```python
from build123d import *

# Parameters (mm, degrees)
CROQUIS1_W              = 192.96
CROQUIS1_H              = 110.76
CROQUIS1_W_2            = 172.96
CROQUIS1_H_2            = 102.76
SALIENTE_EXTRUIR2_DEPTH = 18
CROQUIS2_W              = 31.89
CROQUIS2_H              = 3
SALIENTE_EXTRUIR3_DEPTH = 24.43
CROQUIS3_W              = 31.89
CROQUIS3_H              = 3
SALIENTE_EXTRUIR4_DEPTH = 22.43
CROQUIS1_2_W            = 192.96
CROQUIS1_2_H            = 110.76
CROQUIS1_2_W_2          = 172.96
CROQUIS1_2_H_2          = 102.76
SALIENTE_EXTRUIR5_DEPTH = 22
CROQUIS6_R              = 6.63
SALIENTE_EXTRUIR6_DEPTH = 22
CROQUIS7_R              = 1.55
CORTAR_EXTRUIR1_DEPTH   = 22
CORTAR_EXTRUIR2_DEPTH   = 4
REDONDEO1_R             = 7.88
REDONDEO2_R             = 7.88
REDONDEO3_R             = 7.88
REDONDEO4_R             = 7.88
CROQUIS9_R              = 1.55
CORTAR_EXTRUIR3_DEPTH   = 4
CROQUIS10_W             = 172.96
CROQUIS10_H             = 102.76
CORTAR_EXTRUIR5_DEPTH   = 7.8
REDONDEO5_R             = 7
REDONDEO6_R             = 7
REDONDEO7_R             = 7
REDONDEO8_R             = 7
CROQUIS11_W             = 80
CROQUIS11_H             = 1.5
CORTAR_EXTRUIR6_DEPTH   = 7.8
REDONDEO9_R             = 1.5


with BuildPart() as part:
    # Croquis1 → Saliente-Extruir2 (new body)
    with BuildSketch(Plane(origin=(0, 0, 0), x_dir=(1, 0, 0), z_dir=(0, 1, 0))):
        with Locations((96.48, 55.38)):
            Rectangle(CROQUIS1_W, CROQUIS1_H)
        with Locations((96.48, 54.38)):
            Rectangle(CROQUIS1_W_2, CROQUIS1_H_2, mode=Mode.SUBTRACT)
    extrude(amount=SALIENTE_EXTRUIR2_DEPTH)

    # Croquis2 → Saliente-Extruir3 (add)
    with BuildSketch(Plane(origin=(0, 0, -3), x_dir=(-1, 0, 0), z_dir=(0, 0, -1))):
        with Locations((-25.945, 9.3)):
            Rectangle(CROQUIS2_W, CROQUIS2_H)
        with Locations((-167.015, 9.3)):
            Rectangle(CROQUIS2_W, CROQUIS2_H)
    extrude(amount=SALIENTE_EXTRUIR3_DEPTH)

    # Croquis3 → Saliente-Extruir4 (add)
    with BuildSketch(Plane.XY.offset(-105.76)):
        with Locations((167.015, 9.3)):
            Rectangle(CROQUIS3_W, CROQUIS3_H)
        with Locations((25.945, 9.3)):
            Rectangle(CROQUIS3_W, CROQUIS3_H)
    extrude(amount=SALIENTE_EXTRUIR4_DEPTH)

    # Croquis1<2> → Saliente-Extruir5 (add)
    with BuildSketch(Plane(origin=(0, 0, 0), x_dir=(1, 0, 0), z_dir=(0, 1, 0))):
        with Locations((96.48, 55.38)):
            Rectangle(CROQUIS1_2_W, CROQUIS1_2_H)
        with Locations((96.48, 54.38)):
            Rectangle(CROQUIS1_2_W_2, CROQUIS1_2_H_2, mode=Mode.SUBTRACT)
    extrude(amount=SALIENTE_EXTRUIR5_DEPTH)

    # Croquis6 → Saliente-Extruir6 (add)
    with BuildSketch(Plane(origin=(0, 22, 0), x_dir=(1, 0, 0), z_dir=(0, 1, 0))):
        with Locations((6.63, 6.63)):
            Circle(CROQUIS6_R)
        with Locations((6.63, 104.13)):
            Circle(CROQUIS6_R)
        with Locations((186.33, 104.13)):
            Circle(CROQUIS6_R)
        with Locations((186.33, 6.63)):
            Circle(CROQUIS6_R)
    extrude(amount=-SALIENTE_EXTRUIR6_DEPTH)

    # Croquis7 → Cortar-Extruir1 (cut)
    with BuildSketch(Plane(origin=(0, 22, 0), x_dir=(1, 0, 0), z_dir=(0, 1, 0))):
        with Locations(Location((6.63, 104.13, 0), (0, 0, 270))):
            Circle(CROQUIS7_R)
        with Locations(Location((186.33, 104.13, 0), (0, 0, 270))):
            Circle(CROQUIS7_R)
        with Locations(Location((186.33, 6.63, 0), (0, 0, 270))):
            Circle(CROQUIS7_R)
        with Locations(Location((6.63, 6.63, 0), (0, 0, 270))):
            Circle(CROQUIS7_R)
    extrude(amount=-CORTAR_EXTRUIR1_DEPTH, mode=Mode.SUBTRACT)

    # Croquis8 → Cortar-Extruir2 (cut)
    with BuildSketch(Plane(origin=(0, 22, 0), x_dir=(1, 0, 0), z_dir=(0, 1, 0))):
        Polygon((189.534293994, 6.63), (187.932146997, 9.405), (184.727853003, 9.405), (183.125706006, 6.63), (184.727853003, 3.855), (187.932146997, 3.855), align=None)
        Polygon((189.534293994, 104.13), (187.932146997, 106.905), (184.727853003, 106.905), (183.125706006, 104.13), (184.727853003, 101.355), (187.932146997, 101.355), align=None)
        Polygon((9.834293994, 6.63), (8.232146997, 9.405), (5.027853003, 9.405), (3.425706006, 6.63), (5.027853003, 3.855), (8.232146997, 3.855), align=None)
        Polygon((9.834293994, 104.13), (8.232146997, 106.905), (5.027853003, 106.905), (3.425706006, 104.13), (5.027853003, 101.355), (8.232146997, 101.355), align=None)
    extrude(amount=-CORTAR_EXTRUIR2_DEPTH, mode=Mode.SUBTRACT)

    # Redondeo1
    redondeo1_edges = [part.edges().sort_by_distance(p)[0] for p in [
        (0, 11, 0),
    ]]
    fillet(redondeo1_edges, radius=REDONDEO1_R)

    # Redondeo2
    redondeo2_edges = [part.edges().sort_by_distance(p)[0] for p in [
        (0, 11, -110.76),
    ]]
    fillet(redondeo2_edges, radius=REDONDEO2_R)

    # Redondeo3
    redondeo3_edges = [part.edges().sort_by_distance(p)[0] for p in [
        (192.96, 11, -110.76),
    ]]
    fillet(redondeo3_edges, radius=REDONDEO3_R)

    # Redondeo4
    redondeo4_edges = [part.edges().sort_by_distance(p)[0] for p in [
        (192.96, 11, 0),
    ]]
    fillet(redondeo4_edges, radius=REDONDEO4_R)

    # Croquis9 → Cortar-Extruir3 (cut)
    with BuildSketch(Plane.XZ.offset(-7.8)):
        with Locations((158.09, -89.18)):
            Circle(CROQUIS9_R)
        with Locations((158.09, -23.53)):
            Circle(CROQUIS9_R)
        with Locations((31.89, -89.18)):
            Circle(CROQUIS9_R)
        with Locations((31.89, -23.53)):
            Circle(CROQUIS9_R)
    extrude(amount=-CORTAR_EXTRUIR3_DEPTH, mode=Mode.SUBTRACT)

    # Croquis10 → Cortar-Extruir5 (cut)
    with BuildSketch(Plane.XZ):
        with Locations((96.48, -54.38)):
            Rectangle(CROQUIS10_W, CROQUIS10_H)
    extrude(amount=-CORTAR_EXTRUIR5_DEPTH, mode=Mode.SUBTRACT)

    # Redondeo5
    redondeo5_edges = [part.edges().sort_by_distance(p)[0] for p in [
        (151.07, 9.3, -27.43),
    ]]
    fillet(redondeo5_edges, radius=REDONDEO5_R)

    # Redondeo6
    redondeo6_edges = [part.edges().sort_by_distance(p)[0] for p in [
        (151.07, 9.3, -83.33),
    ]]
    fillet(redondeo6_edges, radius=REDONDEO6_R)

    # Redondeo7
    redondeo7_edges = [part.edges().sort_by_distance(p)[0] for p in [
        (41.89, 9.3, -83.33),
    ]]
    fillet(redondeo7_edges, radius=REDONDEO7_R)

    # Redondeo8
    redondeo8_edges = [part.edges().sort_by_distance(p)[0] for p in [
        (41.89, 9.3, -27.43),
    ]]
    fillet(redondeo8_edges, radius=REDONDEO8_R)

    # Croquis11 → Cortar-Extruir6 (cut)
    with BuildSketch(Plane(origin=(0, 0, 0), x_dir=(-1, 0, 0), z_dir=(0, -1, 0))):
        with Locations((-96.48, 2.25)):
            Rectangle(CROQUIS11_W, CROQUIS11_H)
    extrude(amount=-CORTAR_EXTRUIR6_DEPTH, mode=Mode.SUBTRACT)

    # Redondeo9
    redondeo9_edges = [part.edges().sort_by_distance(p)[0] for p in [
        (96.48, 7.8, -1.5),
    ]]
    fillet(redondeo9_edges, radius=REDONDEO9_R - 0.0001)  # a hair under: the kernel refuses the full size


solid = part.part
```
Here's how the part is built. I have some questions about the finished solid (model axes, mm). A direction names the side the tool comes from. Give positions to 0.01 mm unless a question says otherwise; leave off trailing zeros. Loops run counter-clockwise (first coordinate to the right, second up) from the corner with the lowest first, then second, coordinate; pieces in that order, holes last. Notation, with made-up numbers: M -20.75,25 L 27.25,25 A26 cw 27.25,58 Z; hole C 72.5,-4 d7. An arc over 180 degrees is marked long. Return JSON: item names as keys, results as strings.
Item 1: Thinking about a two-plate mould opening in Z: for faces 1 (the cylindrical face through (179.89, 16.48, -8.21)), 2 (the flat face through (96, 0, -109)), 3 (the cylindrical face through (190.59, 10.846, -108.513)), which applies, released by +Z, released by -Z, zero draft, split by the parting line, or undercut?
A:
{"face 1": "undercut", "face 2": "zero draft", "face 3": "released by -Z"}
Item 2: I'm going to push flat-ended pins straight in: pin 1 Ø3 at (x, z) = (31.89, -23.53) entering from -Y; pin 2 Ø1 at (x, y) = (187, 19.5) entering from +Z; pin 3 Ø4 at (x, z) = (40.5, -91) entering from -Y; pin 4 Ø6.5 at (x, z) = (21, -98.5) entering from +Y. Where does each tip first touch, or does it pass through?
A:
{"pin 1": "passes through", "pin 2": "stops at z = -0.13", "pin 3": "stops at y = 7.8", "pin 4": "stops at y = 10.8"}
Item 3: Imagine slicing it at A-A on z = -61. List the corners of the cut face in (x, y) for me.
A:
{"outline": "M 0,0 L 10,0 L 10,22 L 0,22 Z; M 182.96,0 L 192.96,0 L 192.96,22 L 182.96,22 Z"}
Item 4: Imagine slicing it at B-B on x = 48. List the corners of the cut face in (y, z) for me.
A:
{"outline": "M 0,-110.76 L 22,-110.76 L 22,-105.76 L 0,-105.76 Z; M 0,-3 L 22,-3 L 22,0 L 0,0 Z"}
Item 5: Imagine slicing it at C-C on x = 22. List the corners of the cut face in (y, z) for me, then the cut area to 3 significant figures.
A:
{"outline": "M 0,-110.76 L 22,-110.76 L 22,-105.76 L 10.8,-105.76 L 10.8,-83.33 L 7.8,-83.33 L 7.8,-105.76 L 0,-105.76 Z; M 0,-3 L 7.8,-3 L 7.8,-27.43 L 10.8,-27.43 L 10.8,-3 L 22,-3 L 22,0 L 0,0 Z", "area": "317 mm^2"}
Item 6: Please list where these lines run through material, in increasing order: line 1 (Z direction, x = 158.09, y = 9.1); line 2 (X direction, y = 8.25, z = -9.5); line 3 (X direction, y = 16, z = -24).
A:
{"line 1": "z = -110.76 to -90.73, -87.63 to -83.33, -27.43 to -25.08, -21.98 to 0", "line 2": "x = 0 to 41.89, 151.07 to 192.96", "line 3": "x = 0 to 10, 182.96 to 192.96"}
Item 7: On a 3-axis mill with a long thin cutter (end or side, diameter ignored), from which of +Z, -Z, +X, -X, +Y, -Y can I reach the whole of each face in a straight line? I mean faces 4 (the cylindrical face through (39.89, 9.32, -85.43)), 5 (the flat face through (95, 11, -105.76)), 6 (the flat face through (26, 10.8, -95)), 7 (the flat face through (26, 7.8, -95)). Say none if no direction works.
A:
{"face 4": "+Y, -Y", "face 5": "none", "face 6": "+Y", "face 7": "-Y"}
